Autodesk Inventor part; units mm, degrees
ref_plane "YZ Plane" through (0, 0, 0) normal (1, 0, 0) x (0, 1, 0)
ref_plane "XZ Plane" through (0, 0, 0) normal (0, 1, 0) x (-1, 0, 0)
ref_plane "XY Plane" through (0, 0, 0) normal (0, 0, 1) x (1, 0, 0)
ref_plane "Work Plane1" through (0, 0, 0) normal (0, 0, 1) x (1, 0, 0)
sketch "Sketch1" plane through (0, 0, 0) normal (0, 0, 1) x (1, 0, 0)
  line L0 (-320.6659, 365.07) -> (-303.6236, 365.07)
  spline S0 degree 3 poles (-320.9918, 365.6066) (-321.0765, 365.7292) (-320.8908, 365.3877) (-320.6659, 365.07) knots 2.320993 2.320993 2.320993 2.320993 3 3 3 3
  spline S1 degree 3 poles (-352.5793, 368.487) (-340.4491, 375.5323) (-326.8416, 374.8317) (-320.9918, 365.6066) knots 3 3 3 3 3.981304 3.981304 3.981304 3.981304
  spline S2 degree 3 poles (-366.293, 340.5724) (-371.0762, 348.8109) (-364.9349, 361.3096) (-352.5793, 368.487) knots 4 4 4 4 5 5 5 5
  spline S3 degree 3 poles (-335.2478, 338.6495) (-347.6077, 331.4693) (-361.5095, 332.3307) (-366.293, 340.5724) knots 5 5 5 5 6 6 6 6
  line L1 (-330.2832, 342.0297) -> (-335.2478, 338.6495)
  line L2 (-316.9989, 342.0297) -> (-330.2832, 342.0297)
  line L3 (-327.0734, 324.5796) -> (-316.9989, 342.0297)
  line L4 (-389.8551, 324.5796) -> (-327.0734, 324.5796)
  line L5 (-391.6641, 325.7587) -> (-389.8551, 324.5796)
  line L6 (-399.6179, 339.5077) -> (-391.6641, 325.7587)
  line L7 (-391.0968, 354.2667) -> (-399.6179, 339.5077)
  spline S4 degree 3 poles (-390.4692, 354.2806) (-390.3206, 354.2927) (-390.7092, 354.3026) (-391.0968, 354.2667) knots 2.320993 2.320993 2.320993 2.320993 3 3 3 3
  spline S5 degree 3 poles (-372.1809, 380.196) (-372.1446, 366.1683) (-379.5551, 354.7342) (-390.4692, 354.2806) knots 3 3 3 3 3.981304 3.981304 3.981304 3.981304
  spline S6 degree 3 poles (-389.4988, 406.0297) (-379.9724, 406.0529) (-372.2189, 394.485) (-372.1809, 380.196) knots 4 4 4 4 5 5 5 5
  spline S7 degree 3 poles (-406.6867, 380.1052) (-406.725, 394.3993) (-399.028, 406.008) (-389.4988, 406.0297) knots 5 5 5 5 6 6 6 6
  line L8 (-406.2417, 374.1157) -> (-406.6867, 380.1052)
  line L9 (-412.8838, 362.6111) -> (-406.2417, 374.1157)
  line L10 (-422.9588, 380.0609) -> (-412.8838, 362.6111)
  line L11 (-391.568, 434.4315) -> (-422.9588, 380.0609)
  line L12 (-389.6423, 435.4086) -> (-391.568, 434.4315)
  line L13 (-373.7584, 435.4223) -> (-389.6423, 435.4086)
  line L14 (-365.2373, 420.6633) -> (-373.7584, 435.4223)
  spline S8 degree 3 poles (-365.5391, 420.1128) (-365.6029, 419.9781) (-365.4, 420.3097) (-365.2373, 420.6633) knots 2.320993 2.320993 2.320993 2.320993 3 3 3 3
  spline S9 degree 3 poles (-352.2398, 391.317) (-364.4063, 398.2994) (-370.6033, 410.4341) (-365.5391, 420.1128) knots 3 3 3 3 3.981304 3.981304 3.981304 3.981304
  spline S10 degree 3 poles (-321.2082, 393.3979) (-325.9513, 385.1362) (-339.8462, 384.2054) (-352.2398, 391.317) knots 4 4 4 4 5 5 5 5
  spline S11 degree 3 poles (-335.0655, 421.2453) (-322.6673, 414.1314) (-316.4624, 401.6613) (-321.2082, 393.3979) knots 5 5 5 5 6 6 6 6
  line L15 (-340.4751, 423.8546) -> (-335.0655, 421.2453)
  line L16 (-347.1173, 435.3592) -> (-340.4751, 423.8546)
  line L17 (-326.9678, 435.3595) -> (-347.1173, 435.3592)
  line L18 (-295.577, 380.9889) -> (-326.9678, 435.3595)
  line L19 (-295.6936, 378.8327) -> (-295.577, 380.9889)
  line L20 (-303.6236, 365.07) -> (-295.6936, 378.8327)
  line L21 (-427.984, 366.6864) -> (-429.2569, 380)
  line L22 (-441.4092, 343.8238) -> (-427.984, 366.6864)
  line L23 (-435.1382, 332.0107) -> (-441.4092, 343.8238)
  line L24 (-408.6792, 330.3208) -> (-435.1382, 332.0107)
  line L25 (-398.3649, 321.8068) -> (-408.6792, 330.3208)
  line L26 (-391.6916, 296.1474) -> (-398.3649, 321.8068)
  line L27 (-378.9043, 292.2286) -> (-391.6916, 296.1474)
  line L28 (-359, 309.7431) -> (-378.9043, 292.2286)
  line L29 (-345.6864, 311.016) -> (-359, 309.7431)
  line L30 (-322.8238, 297.5908) -> (-345.6864, 311.016)
  line L31 (-311.0107, 303.8618) -> (-322.8238, 297.5908)
  line L32 (-309.3208, 330.3208) -> (-311.0107, 303.8618)
  line L33 (-300.8068, 340.6351) -> (-309.3208, 330.3208)
  line L34 (-275.1474, 347.3084) -> (-300.8068, 340.6351)
  line L35 (-271.2286, 360.0957) -> (-275.1474, 347.3084)
  line L36 (-288.7431, 380) -> (-271.2286, 360.0957)
  line L37 (-290.016, 393.3136) -> (-288.7431, 380)
  line L38 (-276.5908, 416.1762) -> (-290.016, 393.3136)
  line L39 (-282.8618, 427.9893) -> (-276.5908, 416.1762)
  line L40 (-309.3208, 429.6792) -> (-282.8618, 427.9893)
  line L41 (-319.6351, 438.1932) -> (-309.3208, 429.6792)
  line L42 (-326.3084, 463.8526) -> (-319.6351, 438.1932)
  line L43 (-339.0957, 467.7714) -> (-326.3084, 463.8526)
  line L44 (-359, 450.2569) -> (-339.0957, 467.7714)
  line L45 (-372.3136, 448.984) -> (-359, 450.2569)
  line L46 (-395.1762, 462.4092) -> (-372.3136, 448.984)
  line L47 (-406.9893, 456.1382) -> (-395.1762, 462.4092)
  line L48 (-408.6792, 429.6792) -> (-406.9893, 456.1382)
  line L49 (-417.1932, 419.3649) -> (-408.6792, 429.6792)
  line L50 (-442.8526, 412.6916) -> (-417.1932, 419.3649)
  line L51 (-446.7714, 399.9043) -> (-442.8526, 412.6916)
  line L52 (-429.2569, 380) -> (-446.7714, 399.9043)
  point P0 (0, 0)
extrude "Extrusion1" add sketch "Sketch1" against normal blind 4
properties part number "logoDraw" material "Wood (Cherry)"
The listing builds one solid part. Answer for the finished solid, in the listing's coordinates (mm). A direction names the side the tool comes from. Give positions to 0.01 mm unless a question says otherwise; leave off trailing zeros. Order: outer loops, then holes, each group sorted by start corner. A loop starts at its lowest first (then second) coordinate and runs counter-clockwise, first axis right, second up. Notation, with made-up numbers: (-5, -25.75) - (5, -25.75) arc R27 cw to (5, -0.75) - close; hole circle Ø10 at (35.25, -27). An arc over 180 degrees is marked (long way). Use one line per item in the form item = value.
1) Consider probe 1 along Y at (x, z) = (-391, -2.3); probe 2 along Y at (x, z) = (-360, -1.3); probe 3 along X at (y, z) = (398, -0.2). Determine where each line is inside the solid, lowest interval first. Write a range as [from, to].
Verdict:
probe_1 = [295.94, 325.33], [354.27, 405.93], [434.72, 459.96]
probe_2 = [308.86, 324.58], [335.24, 362.87], [397.24, 450.16]
probe_3 = [-445.1, -412.6], [-401.95, -376.97], [-360.73, -319.71], [-305.4, -287.26]
2) Find section A-A on y = 317.5. Determine the outline of the cut face in (x, z), and give its area (3 significant figures).
Verdict:
outline = (-397.24, -4) - (-310.14, -4) - (-310.14, 0) - (-397.24, 0) - close
area = 348 mm^2
3) For faces 4 (the flat face through (-368.81, 301.11, -1.97)), 5 (the flat face through (-280.11, 370.19, -1.97)), 6 (the flat face through (-383.905, 455.791, -1.972)), 7 (the flat face through (-359, 324.58, -2)), determine the directions among +Z, -Z, +X, -X, +Y, -Y from which every point of the face is accessible in a straight line to the end or side of a thin tool.
Verdict:
face_4 = +Z, -Z, -Y
face_5 = +Z, -Z, +X
face_6 = +Z, -Z, +Y
face_7 = +Z, -Z
4) Each of these flat-tipped pins is pushed along its axis until it touches: pin 1 (2 mm diameter, centred on x = -322.5, z = -3, fed in from -Y); pin 2 (2 mm diameter, centred on x = -340.5, z = -3, fed in from -Y); pin 3 (2 mm diameter, centred on y = 326, z = -3, fed in from +X). Where does it stop, or does it pass through?
Verdict:
pin_1 = 297.59
pin_2 = 307.38
pin_3 = -309.53
5) The mould has two halves that part along Y. Classify faces 1 (the flat face through (-394.982, 308.797, -1.972)), 2 (the flat face through (-428.61, 373.25, -1.97)), 3 (the flat face through (-314.55, 433.996, -1.972)): released by +Y, released by -Y, zero draft, split by the parting line, or undercut.
Verdict:
face_1 = released by -Y
face_2 = undercut
face_3 = released by +Y
